Geometry: final body of the model. Coordinates: model frame, mm. A direction names the side the tool comes from. Give positions to 0.01 mm unless a question says otherwise; leave off trailing zeros. Loops run counter-clockwise (first coordinate to the right, second up) from the corner with the lowest first, then second, coordinate; pieces in that order, holes last. Notation, with made-up numbers: (-29.75, 24.25) -> (-8.75, 24.25) arc R19 ccw to (-8.75, 38.25) -> close; hole circle Ø4 at (57, 47). An arc over 180 degrees is marked (long way). Answer in a Markdown table with one row per item. Add a question column.
from build123d import *

# Parameters (mm, degrees)
F1_DEPTH = 2
F2_DEPTH = 10


with BuildPart() as f1:
    # F0 (on Top) → F1 (new body)
    with BuildSketch(Plane.XY):
        with BuildLine():
            Line((4, 14.456832), (4, 0))
            ThreePointArc((4, 0), (0, -4), (-4, 0))
            Line((-4, 0), (-4, 14.456832))
            ThreePointArc((-4, 14.456832), (-9.082951, -11.937336), (15, 0))
            ThreePointArc((15, 0), (11.937336, 9.082951), (4, 14.456832))
        make_face()
        with BuildLine():
            ThreePointArc((-4, 0), (0, 4), (4, 0))
            Line((4, 0), (4, 14.456832))
            ThreePointArc((4, 14.456832), (0, 15), (-4, 14.456832))
            Line((-4, 14.456832), (-4, 0))
        make_face()
        with BuildLine():
            ThreePointArc((-4, 0), (0, -4), (4, 0))
            ThreePointArc((4, 0), (0, 4), (-4, 0))
        make_face()
    extrude(amount=F1_DEPTH)

    # F0 (on Top) → F2 (join)
    with BuildSketch(Plane.XY):
        with BuildLine():
            Line((4, 14.456832), (4, 0))
            ThreePointArc((4, 0), (0, -4), (-4, 0))
            Line((-4, 0), (-4, 14.456832))
            ThreePointArc((-4, 14.456832), (-9.082951, -11.937336), (15, 0))
            ThreePointArc((15, 0), (11.937336, 9.082951), (4, 14.456832))
        make_face()
    extrude(amount=F2_DEPTH)


solid = f1.part
(1) Draft query along X for faces 3 (the flat face through (3, -3, 10)), 4 (the flat face through (4, 7, 6)). Return one class per face: +X half, -X half, draft (parallel to the pull), parting line (faces both ways), or undercut.
(2) Cut plane A-A on z = 6.25. Return the cut outline in (x, y), then the cut area to 3 significant figures.
(3) Reachability of faces 1 (the cylindrical face through (0, -4, 6)), 2 (the flat face through (0, 0, 0)) from +Z, -Z, +X, -X, +Y, -Y: full face, straight path, thin tool, end or side. Return the list, or none.
(4) Cut plane C-C on y = 6.5. Return the cut outline in (x, z), then the cut area to 3 significant figures.
(5) Pin query (flat end, axial travel): pin 1 Ø4 at (x, z) = (-11, 1) entering from +Y; pin 2 Ø1.5 at (x, z) = (0, 6) entering from +Y; pin 3 Ø2.5 at (y, z) = (6, 5) entering from -X. Return the tip coordinate at first contact, or that it passes through.
(6) Cut plane B-B on x = 0. Return the cut outline in (y, z), then the cut area to 3 significant figures.
(7) Material intervals for line 1 along X through (y, z) = (-0.25, 4.75); line 2 along X through (y, z) = (12, 3.75); line 3 along X through (y, z) = (-9.75, 2.5), sorted ascending. Write a range as from..to.
(8) Cut plane D-D on z = 1. Return the cut outline in (x, y).
Answer list:
| question | item | result |
|---|---|---|
| 1 | face 3 | draft |
| 1 | face 4 | undercut |
| 2 | outline | (-4, 0) -> (-4, 14.46) arc R15 ccw (long way) to (4, 14.46) -> (4, 0) arc R4 cw to start |
| 2 | area | 563 mm² |
| 3 | face 1 | +Z, +Y |
| 3 | face 2 | -Z, +X, -X, +Y, -Y |
| 4 | outline | (-13.52, 0) -> (13.52, 0) -> (13.52, 10) -> (4, 10) -> (4, 2) -> (-4, 2) -> (-4, 10) -> (-13.52, 10) -> close |
| 4 | area | 206 mm² |
| 5 | pin 1 | stops at y = 12 |
| 5 | pin 2 | stops at y = -3.93 |
| 5 | pin 3 | stops at x = -14.23 |
| 6 | outline | (-15, 0) -> (15, 0) -> (15, 2) -> (-4, 2) -> (-4, 10) -> (-15, 10) -> close |
| 6 | area | 148 mm² |
| 7 | line 1 | x = -15..-3.99, 3.99..15 |
| 7 | line 2 | x = -9..-4, 4..9 |
| 7 | line 3 | x = -11.4..11.4 |
| 8 | outline | (-4, 14.46) arc R15 ccw (long way) to (4, 14.46) arc R15 ccw to start |
